Geometry check sheet. Reference: the model listing, model coordinates, mm. A direction names the side the tool comes from. Give positions to 0.01 mm unless a question says otherwise; leave off trailing zeros. Write each loop counter-clockwise with the first axis right and the second up, starting at its lowest first coordinate (ties: lowest second). Pieces come first, ordered by that corner, then holes. Notation, with made-up numbers: (42, -22.75) -> (58, -22.75) arc R19 ccw to (58, 5.25) -> close; hole circle Ø2 at (50.25, 17.5). An arc over 180 degrees is marked (long way). One line per item, written item: value.
from build123d import *

# Parameters (mm, degrees)
SKETCH1_W           = 31.75
SKETCH1_H           = 35.814
BOSS_EXTRUDE1_DEPTH = 10.16
SKETCH3_R           = 11
BOSS_EXTRUDE2_DEPTH = 14.478
SKETCH4_W           = 16
SKETCH4_H           = 5.5
BOSS_EXTRUDE3_DEPTH = 15.24
SKETCH5_R           = 9.5
CUT_EXTRUDE1_DEPTH  = 8.5
SKETCH6_R           = 2
CUT_EXTRUDE2_DEPTH  = 8.5
SKETCH7_R           = 2
CUT_EXTRUDE3_DEPTH  = 8.5
SKETCH8_W           = 12
SKETCH8_H           = 1.6
CUT_EXTRUDE4_DEPTH  = 15.15
SKETCH10_W          = 12
SKETCH10_H          = 1.6
CUT_EXTRUDE5_DEPTH  = 15.15
SKETCH12_R          = 4.135780917
BOSS_EXTRUDE4_DEPTH = 15.15
SKETCH13_R          = 3
CUT_EXTRUDE6_DEPTH  = 15.15
SKETCH14_R          = 4.135
BOSS_EXTRUDE5_DEPTH = 15.15
SKETCH15_R          = 3
CUT_EXTRUDE7_DEPTH  = 15.15


with BuildPart() as part:
    # Sketch1 → Boss-Extrude1 (new body)
    with BuildSketch(Plane.XY):
        Rectangle(SKETCH1_W, SKETCH1_H)
    extrude(amount=BOSS_EXTRUDE1_DEPTH)

    # Sketch3 → Boss-Extrude2 (add)
    with BuildSketch(Plane.XY.offset(10.16)):
        with Locations((-0.024824202, 1.289107608)):
            Circle(SKETCH3_R)
    extrude(amount=BOSS_EXTRUDE2_DEPTH)

    # Sketch4 → Boss-Extrude3 (add)
    with BuildSketch(Plane(origin=(0, 0, 0), x_dir=(-1, 0, 0), z_dir=(0, 0, -1))):
        Rectangle(SKETCH4_W, SKETCH4_H)
    extrude(amount=BOSS_EXTRUDE3_DEPTH)

    # Sketch5 → Cut-Extrude1 (cut)
    with BuildSketch(Plane.XY.offset(24.638)):
        with Locations((0, 1.039705526)):
            Circle(SKETCH5_R)
        with BuildLine():
            Line((-8.015794219, 0), (8.518877538, 0))
            ThreePointArc((8.518877538, 0), (0.25154166, -7.404071177), (-8.015794219, 0))
        make_face(mode=Mode.SUBTRACT)
        with BuildLine():
            Line((-8.015794219, 1.039705526), (8.518877538, 1.039705526))
            ThreePointArc((8.518877538, 1.039705526), (0.25154166, 9.706845425), (-8.015794219, 1.039705526))
        make_face(mode=Mode.SUBTRACT)
    extrude(amount=-CUT_EXTRUDE1_DEPTH, mode=Mode.SUBTRACT)

    # Sketch6 → Cut-Extrude2 (cut)
    with BuildSketch(Plane.XY.offset(24.638)):
        with Locations((0, 5.366222071)):
            Circle(SKETCH6_R)
    extrude(amount=-CUT_EXTRUDE2_DEPTH, mode=Mode.SUBTRACT)

    # Sketch7 → Cut-Extrude3 (cut)
    with BuildSketch(Plane.XY.offset(24.638)):
        with Locations((0, -3.488044346)):
            Circle(SKETCH7_R)
    extrude(amount=-CUT_EXTRUDE3_DEPTH, mode=Mode.SUBTRACT)

    # Sketch8 → Cut-Extrude4 (cut)
    with BuildSketch(Plane(origin=(0, 0, -15.24), x_dir=(-1, 0, 0), z_dir=(0, 0, -1))):
        with Locations((0, 1.95)):
            Rectangle(SKETCH8_W, SKETCH8_H)
    extrude(amount=-CUT_EXTRUDE4_DEPTH, mode=Mode.SUBTRACT)

    # Sketch10 → Cut-Extrude5 (cut)
    with BuildSketch(Plane(origin=(0, 0, -15.24), x_dir=(-1, 0, 0), z_dir=(0, 0, -1))):
        with Locations((0, -1.95)):
            Rectangle(SKETCH10_W, SKETCH10_H)
    extrude(amount=-CUT_EXTRUDE5_DEPTH, mode=Mode.SUBTRACT)

    # Sketch12 → Boss-Extrude4 (add)
    with BuildSketch(Plane(origin=(0, 0, 0), x_dir=(-1, 0, 0), z_dir=(0, 0, -1))):
        with Locations((0, 5.523554626)):
            Circle(SKETCH12_R)
    extrude(amount=BOSS_EXTRUDE4_DEPTH)

    # Sketch13 → Cut-Extrude6 (cut)
    with BuildSketch(Plane(origin=(0, 0, -15.15), x_dir=(-1, 0, 0), z_dir=(0, 0, -1))):
        with Locations((0, 5.628086678)):
            Circle(SKETCH13_R)
    extrude(amount=-CUT_EXTRUDE6_DEPTH, mode=Mode.SUBTRACT)

    # Sketch14 → Boss-Extrude5 (add)
    with BuildSketch(Plane(origin=(0, 0, 0), x_dir=(-1, 0, 0), z_dir=(0, 0, -1))):
        with Locations((0, -5.366222071)):
            Circle(SKETCH14_R)
    extrude(amount=BOSS_EXTRUDE5_DEPTH)

    # Sketch15 → Cut-Extrude7 (cut)
    with BuildSketch(Plane(origin=(0, 0, -15.15), x_dir=(-1, 0, 0), z_dir=(0, 0, -1))):
        with Locations((0, -5.366222071)):
            Circle(SKETCH15_R)
    extrude(amount=-CUT_EXTRUDE7_DEPTH, mode=Mode.SUBTRACT)


solid = part.part
1) Depth check by flat-ended pin: pin 1 Ø6 at (x, y) = (4, -13.5) entering from -Z; pin 2 Ø6.5 at (x, y) = (-1.5, 6) entering from -Z; pin 3 Ø1 at (y, z) = (-8, 20.5) entering from +X. Enter the tip coordinate at first touch or a pass-through.
Verdict:
pin 1: z = 0
pin 2: z = -15.15
pin 3: x = 6.59
2) Tool access check on faces 1 (the flat face through (1.4, 1.4, -0.09)), 2 (the flat face through (2.5, 3.7, -15.15)), 3 (the flat face through (15.875, 0, 5)), 4 (the flat face through (-7, -8, 10.16)), 5 (the flat face through (0, 17.907, 5)). Record the directions out of +Z, -Z, +X, -X, +Y, -Y that give a thin tool (end or side, any length) a straight path to the whole face; none if there is none.
Verdict:
face 1: -Z
face 2: -Z, +Y
face 3: +Z, -Z, +X, +Y, -Y
face 4: +Z
face 5: +Z, -Z, +X, -X, +Y
3) Sectioned sample at A-A on z = -3.5. Record the cut outline in (x, y) (3 decimals).
Verdict:
outline: (-8, -2.75) -> (-6, -2.75) -> (-6, -1.15) -> (6, -1.15) -> (6, -2.75) -> (8, -2.75) -> (8, 2.75) -> (6, 2.75) -> (6, 1.15) -> (-6, 1.15) -> (-6, 2.75) -> (-8, 2.75) -> close; circle Ø8.272 at (0, 5.524); circle Ø8.27 at (0, -5.366); hole circle Ø6 at (0, -5.366); hole circle Ø6 at (0, 5.628)
4) Sectioned sample at B-B on z = 19.5. Record the cut outline in (x, y), plus the area to 3 significant figures.
Verdict:
outline: circle Ø22 at (-0.02, 1.29); (-8.02, 0) arc R8.32 ccw to (8.52, 0) -> close; (-8.02, 1.04) -> (8.52, 1.04) arc R8.28 ccw (long way) to start; hole circle Ø19 at (0, 1.04); hole circle Ø4 at (0, -3.49); hole circle Ø4 at (0, 5.37)
area: 279 mm^2
5) Sectioned sample at D-D on z = 14. Record the cut outline in (x, y).
Verdict:
outline: circle Ø22 at (-0.02, 1.29)
6) Scan lines: probe 1 along Y at (x, z) = (0, 21); probe 2 along Z at (x, y) = (-3.5, 14.5); probe 3 along X at (y, z) = (8.5, 23). Record each from-to range of solid material in increasing order.
Verdict:
probe 1: -9.71 to -8.46, -7.4 to -5.49, -1.49 to 0, 1.04 to 3.37, 7.37 to 9.7, 10.54 to 12.29
probe 2: 0 to 10.16
probe 3: -8.33 to -5.88, -4.05 to 4.56, 5.88 to 8.28
7) Mould release check, pull along X, two halves, no side actions. Record for faces 6 (the flat face through (-8, 0, -8)), 7 (the flat face through (0, 1.15, -8)), 8 (the flat face through (-3.3, 10.3, 24.638)): released by +X, released by -X, zero draft, split by the parting line, or undercut.
Verdict:
face 6: released by -X
face 7: undercut
face 8: zero draft
8) Sectioned sample at C-C on y = -12. Record the cut outline in (x, z) (3 decimals).
Verdict:
outline: (-15.875, 0) -> (15.875, 0) -> (15.875, 10.16) -> (-15.875, 10.16) -> close
